Read the model definition and answer for the solid it produces. Units are mm, in the model's axes. A direction names the side the tool comes from. Coordinates: 2 decimals unless noted, no trailing zeros. Write each loop counter-clockwise with the first axis right and the second up, starting at its lowest first coordinate (ties: lowest second). Pieces come first, ordered by that corner, then holes.
1) The part is cut by section C-C (x = -60). Determine the outline of the cut face in (y, z), then the cut area to 3 significant figures.
2) The part is cut by section A-A (z = 17.7). Determine the outline of the cut face in (x, y), then the cut area to 3 significant figures.
3) Determine the mould class of faces 1 (the face through (-10, 42, 1)), 2 (the face through (-25, 23, 28)), 3 (the face through (-52.044, 24.294, 2.465)), 4 (the face through (-14.236, 36.224, 0.986)) for opening direction Y: +Y half, -Y half, draft (parallel to the pull), parting line (faces both ways), or undercut.
4) The part is cut by section D-D (y = 32). Determine the outline of the cut face in (x, z).
5) Which of the six approach directions +Z, -Z, +X, -X, +Y, -Y give full straight-line access (tool end or side, diameter ignored) to faces 5 (the face through (-22, 18, 0)), 6 (the face through (-50.916, 22.227, 2.465))?
6) Each of these flat-tipped pins is pushed along its axis until it touches: pin 1 Ø8 at (y, z) = (6.5, 46.5) entering from +X; pin 2 Ø12 at (x, y) = (-14.5, 21) entering from +Z; pin 3 Ø0.7 at (y, z) = (38.5, 1.5) entering from -X; pin 4 Ø3 at (x, y) = (-56, 15.5) entering from +Z. Where does it stop, or does it pass through?
7) The part is cut by section B-B (x = -39.7). Determine the outline of the cut face in (y, z), then the cut area to 3 significant figures.
8) Find the intervals of material crossed by line 1 (X direction, y = 0.8, z = 17.7); line 2 (Y direction, x = -53.5, z = 25.5); line 3 (X direction, y = 40, z = 13), in increasing order.
from build123d import *

# Parameters (mm, degrees)
SKETCH1_W           = 25
SKETCH1_H           = 45
BOSS_EXTRUDE1_DEPTH = 2
SKETCH2_W           = 11
SKETCH2_H           = 6.5
CUT_EXTRUDE1_DEPTH  = 19.78
FILLET1_R           = 2.54
BOSS_EXTRUDE5_DEPTH = 2
SKETCH10_W          = 52.8
SKETCH10_H          = 3
BOSS_EXTRUDE6_DEPTH = 50.8
BOSS_EXTRUDE7_DEPTH = 5
SKETCH12_R          = 6.35
CUT_EXTRUDE4_DEPTH  = 5


with BuildPart() as part:
    # Sketch1 → Boss-Extrude1 (new body)
    with BuildSketch(Plane.XY):
        with Locations((-12.5, 22.5)):
            Rectangle(SKETCH1_W, SKETCH1_H)
    extrude(amount=BOSS_EXTRUDE1_DEPTH)

    # Sketch2 → Cut-Extrude1 (cut)
    with BuildSketch(Plane.XY.offset(2)):
        with Locations((-9.5, 8.25)):
            Rectangle(SKETCH2_W, SKETCH2_H)
        with Locations((-9.5, 38.75)):
            Rectangle(SKETCH2_W, SKETCH2_H)
    extrude(amount=-CUT_EXTRUDE1_DEPTH, mode=Mode.SUBTRACT)

    # Fillet1
    fillet1_edges = [part.edges().sort_by_distance(p)[0] for p in [
        (-15, 11.5, 1),
        (-4, 11.5, 1),
        (-4, 5, 1),
        (-15, 5, 1),
        (-15, 42, 1),
        (-4, 42, 1),
        (-4, 35.5, 1),
        (-15, 35.5, 1),
    ]]
    fillet(fillet1_edges, radius=FILLET1_R)

    # Sketch9 → Boss-Extrude5 (add)
    with BuildSketch(Plane.ZY.offset(25)):
        Polygon((0, 45), (2, 45), (52.8, 45), (52.8, 0), (2, 0), (0, 0), align=None)
    extrude(amount=BOSS_EXTRUDE5_DEPTH)

    # Sketch10 → Boss-Extrude6 (add)
    with BuildSketch(Plane.ZY.offset(27)):
        with Locations((26.4, 1.5)):
            Rectangle(SKETCH10_W, SKETCH10_H)
    extrude(amount=BOSS_EXTRUDE6_DEPTH)

    # Sketch11 → Boss-Extrude7 (add)
    with BuildSketch(Plane(origin=(0, 0, 0), x_dir=(-1, 0, 0), z_dir=(0, 0, -1))):
        Polygon((27, 45), (77.8, 3), (77.8, 0), (27, 42), align=None)
    extrude(amount=-BOSS_EXTRUDE7_DEPTH)

    # Sketch12 → Cut-Extrude4 (cut)
    with BuildSketch(Plane(origin=(0, 3, 0), x_dir=(1, 0, 0), z_dir=(0, 1, 0))):
        with Locations(Location((-39.7, -17.7, 0), (0, 0, 270))):
            Circle(SKETCH12_R)
    extrude(amount=-CUT_EXTRUDE4_DEPTH, mode=Mode.SUBTRACT)


solid = part.part
Reported:
1. outline: (0, 0) - (3, 0) - (3, 52.8) - (0, 52.8) - close; (14.72, 0) - (17.72, 0) - (17.72, 5) - (14.72, 5) - close
1. area: 173 mm2
2. outline: (-77.8, 0) - (-46.05, 0) - (-46.05, 3) - (-77.8, 3) - close; (-33.35, 0) - (-25, 0) - (-25, 45) - (-27, 45) - (-27, 3) - (-33.35, 3) - close
2. area: 204 mm2
3. face 1: undercut
3. face 2: draft
3. face 3: +Y half
3. face 4: undercut
4. outline: (-42.72, 0) - (-39.1, 0) - (-39.1, 5) - (-42.72, 5) - close; (-27, 0) - (0, 0) - (0, 2) - (-25, 2) - (-25, 52.8) - (-27, 52.8) - close
5. face 5: -Z, +X, -X, +Y, -Y
5. face 6: +Z, -Z
6. pin 1: stops at x = -25
6. pin 2: stops at z = 2
6. pin 3: stops at x = -35.29
6. pin 4: passes through
7. outline: (0, 0) - (3, 0) - (3, 11.35) - (0, 11.35) - close; (0, 24.05) - (3, 24.05) - (3, 52.8) - (0, 52.8) - close; (31.5, 0) - (34.5, 0) - (34.5, 5) - (31.5, 5) - close
7. area: 135 mm2
8. line 1: x = -77.8 to -46.05, -33.35 to -25
8. line 2: y = 0 to 3
8. line 3: x = -27 to -25
